from build123d import *

# Parameters (mm, degrees)
F0_R     = 9.652
F0_R_2   = 6.858
F1_DEPTH = 3.302
F2_R     = 9.652
F2_R_2   = 8.001
F3_DEPTH = 7.62
F4_R     = 9.652
F4_R_2   = 8.001
F4_R_3   = 6.858
F5_DEPTH = 8.89
F6_R     = 8.636
F6_R_2   = 6.858
F7_DEPTH = 21.844
F8_R     = 0.88899


# Not quite as in the source:
# - a fillet or chamfer is up to 0.001 mm smaller than in the source, because OpenCascade refuses the exact size


with BuildPart() as f1:
    # F0 (on Front) → F1 (new body)
    with BuildSketch(Plane.XZ):
        Circle(F0_R)
        Circle(F0_R_2, mode=Mode.SUBTRACT)
    extrude(amount=F1_DEPTH)

    # F2 (on face) → F3 (join)
    with BuildSketch(Plane.XZ.offset(3.302)):
        Circle(F2_R)
        Circle(F2_R_2, mode=Mode.SUBTRACT)
    extrude(amount=F3_DEPTH)

    # F4 (on face) → F5 (join)
    with BuildSketch(Plane.XZ.offset(10.922)):
        Circle(F4_R)
        Circle(F4_R_2, mode=Mode.SUBTRACT)
        Circle(F4_R_2)
        Circle(F4_R_3, mode=Mode.SUBTRACT)
    extrude(amount=F5_DEPTH)

    # F6 (on face) → F7 (join)
    with BuildSketch(Plane(origin=(0, 0, 0), x_dir=(-1, 0, 0), z_dir=(0, 1, 0))):
        Circle(F6_R)
        Circle(F6_R_2, mode=Mode.SUBTRACT)
    extrude(amount=F7_DEPTH)

    # F8 (radius 0.889 in the source; OpenCascade refuses exactly that, so slightly less here)
    f8_edges = [f1.edges().sort_by_distance(p)[0] for p in [
        (6.858, 21.844, 0),
        (8.636, 21.844, 0),
    ]]
    fillet(f8_edges, radius=F8_R)


solid = f1.part
CAD build for the part. Positions are in the model's coordinates, mm. A direction names the side the tool comes from. Give positions to 0.01 mm unless a question says otherwise; leave off trailing zeros. Order: outer loops, then holes, each group sorted by start corner. A loop starts at its lowest first (then second) coordinate and runs counter-clockwise, first axis right, second up. Notation, with made-up numbers: (62, -20.75) - (68, -20.75) arc R27 ccw to (68, 5.25) - close; hole circle Ø10 at (6.25, -26.5). An arc over 180 degrees is marked (long way). Answer in a Markdown table with one row per item.
1. Saw through at C-C, the plane y = -6. Give the cut face in (x, z).
Data:
| item | result |
|---|---|
| outline | circle Ø19.3 at (0, 0); hole circle Ø16 at (0, 0) |
2. Tool access for faces 5 (the cylindrical face through (-1.73, -7.06, -7.81)), 6 (the cylindrical face through (1.124, 10.331, 8.563)), 7 (the flat face through (2, -19.812, 7)): list every direction of +Z, -Z, +X, -X, +Y, -Y with a clear straight run to the whole face (end or side of a thin tool).
Data:
| item | result |
|---|---|
| face 5 | none |
| face 6 | +Y |
| face 7 | +Z, -Z, +X, -X, -Y |
3. Probe probe 1 along Z at (x, y) = (0, -18); probe 2 along Z at (x, y) = (0, -6.5); probe 3 along Y at (x, z) = (4.5, 6.25). List the from-to ranges inside material, lowest first. Write a range as [from, to].
Data:
| item | result |
|---|---|
| probe 1 | z = [-9.65, -6.86], [6.86, 9.65] |
| probe 2 | z = [-9.65, -8], [8, 9.65] |
| probe 3 | y = [-19.81, -10.92], [-3.3, 21.84] |
4. Pull direction X, two halves, no side cores. Call faces 1 (the cylindrical face through (-7.66, -9.77, -5.87)), 2 (the flat face through (6, -3.302, 4)), 3 (the flat face through (-1, 0, -9)), 4 (the cylindrical face through (-1.487, -15.305, -6.695)): pulls with the +X half, pulls with the -X half, needs draft (parallel to the pull), parting line crosses it, or undercut.
Data:
| item | result |
|---|---|
| face 1 | parting line crosses it |
| face 2 | undercut |
| face 3 | needs draft |
| face 4 | undercut |
5. Flat gauge pins, fed straight in: pin 1 (1 mm diameter, centred on y = -7, z = 3, fed in from -X); pin 2 (10 mm diameter, centred on x = -7.5, y = -10, fed in from -Z); pin 3 (1 mm diameter, centred on y = -11.5, z = -1.5, fed in from +X). Where does each tip first touch, or does it go through?
Data:
| item | result |
|---|---|
| pin 1 | stops at x = -9.32 |
| pin 2 | stops at z = -9.32 |
| pin 3 | stops at x = 9.6 |
6. Saw through at D-D, the plane y = 9.5. Give the cut face in (x, z), plus the area to 3 significant figures.
Data:
| item | result |
|---|---|
| outline | circle Ø17.27 at (0, 0); hole circle Ø13.72 at (0, 0) |
| area | 86.5 mm² |
